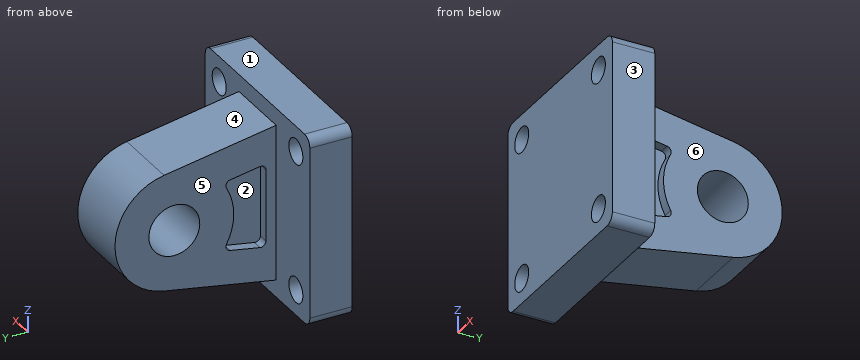
```python
from build123d import *

# Parameters (mm, degrees)
SKETCH_3_W               = 45
SKETCH_3_H               = 45
EXTRUDE_1_DEPTH          = 10
EXTRUDE_START            = -8
EXTRUDE_2_DEPTH          = 16
SKETCH_5_R               = 6
CUT_EXTRUDE_1_DEPTH      = 62.159627206
CUT_EXTRUDE_START        = -2.4
CUT_EXTRUDE_3_DEPTH      = 2.4
SKETCH_7_R               = 3
CUT_EXTRUDE_2_DEPTH      = 50.563091106
MIRROR_2_COPY_1_SKETCH_R = 3
MIRROR_2_COPY_1_DEPTH    = 50.563091106
FILLET_1_R               = 2.25
FILLET_2_R               = 1.2


with BuildPart() as part:
    # 草图3 → 凸台-拉伸1 (new body)
    with BuildSketch(Plane(origin=(0, 0, 0), x_dir=(1, 0, 0), z_dir=(0, 1, 0))):
        Rectangle(SKETCH_3_W, SKETCH_3_H)
    extrude(amount=EXTRUDE_1_DEPTH)

    # 草图4 → 凸台-拉伸2 (add)
    with BuildSketch(Plane(origin=(0, 0, 0), x_dir=(0, 0, -1), z_dir=(1, 0, 0)).offset(EXTRUDE_START)):
        with BuildLine():
            Line((-13.787308542, 36.431074487), (-18.447820103, 10))
            Line((-18.447820103, 10), (18.447820103, 10))
            Line((18.447820103, 10), (13.787308542, 36.431074487))
            ThreePointArc((13.787308542, 36.431074487), (0, 48), (-13.787308542, 36.431074487))
        make_face()
    extrude(amount=EXTRUDE_2_DEPTH)

    # 草图5 → 切除-拉伸1 (cut, through all)
    with BuildSketch(Plane(origin=(8, 0, 0), x_dir=(0, 0, -1), z_dir=(1, 0, 0))):
        with Locations((0, 34)):
            Circle(SKETCH_5_R)
    extrude(amount=-CUT_EXTRUDE_1_DEPTH, mode=Mode.SUBTRACT)

    # 草图8 → 切除-拉伸3 (cut)
    with BuildSketch(Plane(origin=(8, 0, 0), x_dir=(0, 0, -1), z_dir=(1, 0, 0)).offset(CUT_EXTRUDE_START)):
        with BuildLine():
            Line((-8.10534153, 22.584946838), (-9.901222455, 12.4))
            Line((-9.901222455, 12.4), (9.901222455, 12.4))
            Line((9.901222455, 12.4), (8.10534153, 22.584946838))
            ThreePointArc((8.10534153, 22.584946838), (0, 20), (-8.10534153, 22.584946838))
        make_face()
    cut_extrude_3 = extrude(amount=CUT_EXTRUDE_3_DEPTH, mode=Mode.SUBTRACT)

    # 镜向3: 切除-拉伸3 across plane
    add(cut_extrude_3.mirror(Plane(origin=(0, 0, 0), x_dir=(0, 0, 1), z_dir=(1, 0, 0))), mode=Mode.SUBTRACT)

    # 草图7 → 切除-拉伸2 (cut, through all)
    with BuildSketch(Plane(origin=(0, 10, 0), x_dir=(1, 0, 0), z_dir=(0, 1, 0))):
        with Locations(Location((-16.5, 16.5, 0), (0, 0, 270))):
            Circle(SKETCH_7_R)
    cut_extrude_2 = extrude(amount=-CUT_EXTRUDE_2_DEPTH, mode=Mode.SUBTRACT)

    # 镜向1: 切除-拉伸2 across plane
    add(cut_extrude_2.mirror(Plane(origin=(0, 0, 0), x_dir=(0, 0, 1), z_dir=(1, 0, 0))), mode=Mode.SUBTRACT)

    # 镜向2: 切除-拉伸2 across plane
    add(cut_extrude_2.mirror(Plane.XY), mode=Mode.SUBTRACT)

    # 镜向2 copy 1 sketch → 镜向2 copy 1 (cut, through all)
    with BuildSketch(Plane(origin=(0, 10, 0), x_dir=(-1, 0, 0), z_dir=(0, 1, 0))):
        with Locations(Location((-16.5, 16.5, 0), (0, 0, 270))):
            Circle(MIRROR_2_COPY_1_SKETCH_R)
    extrude(amount=-MIRROR_2_COPY_1_DEPTH, mode=Mode.SUBTRACT)

    # 圆角1
    fillet_1_edges = [part.edges().sort_by_distance(p)[0] for p in [
        (-22.5, 5, 22.5),
        (-22.5, 5, -22.5),
        (22.5, 5, -22.5),
        (22.5, 5, 22.5),
    ]]
    fillet(fillet_1_edges, radius=FILLET_1_R)

    # 圆角2
    fillet_2_edges = [part.edges().sort_by_distance(p)[0] for p in [
        (6.8, 22.584946838, 8.10534153),
        (6.8, 22.584946838, -8.10534153),
        (6.8, 12.4, -9.901222455),
        (6.8, 12.4, 9.901222455),
        (-6.8, 22.584946838, -8.10534153),
        (-6.8, 22.584946838, 8.10534153),
        (-6.8, 12.4, 9.901222455),
        (-6.8, 12.4, -9.901222455),
    ]]
    fillet(fillet_2_edges, radius=FILLET_2_R)


solid = part.part
```
Verification items for the finished model (mm, model axes). Face numbers are marked on the shaded views. A direction names the side the tool comes from. Give positions to 0.01 mm unless a question says otherwise; leave off trailing zeros. Order: outer loops, then holes, each group sorted by start corner. A loop starts at its lowest first (then second) coordinate and runs counter-clockwise, first axis right, second up. Notation, with made-up numbers: (81.25, -29.75) - (94.25, -29.75) arc R16 ccw to (94.25, -12.75) - close; hole circle Ø1 at (-11.75, 11.25). An arc over 180 degrees is marked (long way). Answer as CSV lines item,"result". Start each with the question number.
Item 1: Material ranges on L1, parallel to X at y = 6.25, z = 16.5; L2, parallel to Y at x = -3, z = -19, recorded low to high.
Item 2: Section check A-A, the plane x = 16.5. Record the boundary of the cut face in (y, z), plus the area to 3 significant figures.
Item 3: Mould release check, pull along Z, two halves, no side actions. Record for the marked faces 1, 2 and 3: released by +Z, released by -Z, zero draft, split by the parting line, or undercut.
Item 4: Section check D-D, the plane z = -16.5. Record the boundary of the cut face in (x, y).
Item 5: Gauge pin test, flat ends, axial feed: pin 1 (7.5 mm diameter, centred on y = 16, z = 3, fed in from +X); pin 2 (1.9 mm diameter, centred on x = -6.5, z = 1.5, fed in from +Y); pin 3 (1.5 mm diameter, centred on x = -1, y = 25.5, fed in from -Z). Record the tip position at first contact, or that the pin passes through.
Item 6: Section check C-C, the plane x = 7. Record the boundary of the cut face in (y, z), plus the area to 3 significant figures.
Item 7: Section check B-B, the plane y = 7.5. Record the boundary of the cut face in (x, z).
Item 8: Access from +Z, -Z, +X, -X, +Y, -Y to the whole of each face (thin tool, end or side, straight path). Record for the marked faces 4, 5 and 6.
Filled in:
1,L1,"-22.5 to -19.5, -13.5 to 13.5, 19.5 to 22.5"
1,L2,"0 to 10"
2,outline,"(0, -22.5) - (10, -22.5) - (10, -19.5) - (0, -19.5) - close; (0, -13.5) - (10, -13.5) - (10, 13.5) - (0, 13.5) - close; (0, 19.5) - (10, 19.5) - (10, 22.5) - (0, 22.5) - close"
2,area,"330 mm^2"
3,face 1,"released by +Z"
3,face 2,"undercut"
3,face 3,"zero draft"
4,outline,"(-22.5, 0) - (-19.5, 0) - (-19.5, 10) - (-22.5, 10) - close; (-13.5, 0) - (13.5, 0) - (13.5, 10) - (8, 10) - (8, 21.05) - (-8, 21.05) - (-8, 10) - (-13.5, 10) - close; (19.5, 0) - (22.5, 0) - (22.5, 10) - (19.5, 10) - close"
5,pin 1,"x = 8"
5,pin 2,"y = 47.99"
5,pin 3,"z = -15.85"
6,outline,"(0, -22.5) - (10, -22.5) - (10, -18.45) - (36.43, -13.79) arc R14 ccw to (36.43, 13.79) - (10, 18.45) - (10, 22.5) - (0, 22.5) - close; hole (12.4, -8.47) arc R1.2 ccw to (13.81, -9.65) - (20.84, -8.41) arc R1.2 ccw to (21.69, -6.66) arc R14 cw to (21.69, 6.66) arc R1.2 ccw to (20.84, 8.41) - (13.81, 9.65) arc R1.2 ccw to (12.4, 8.47) - close; hole circle Ø12 at (34, 0)"
6,area,"1,280 mm^2"
7,outline,"(-22.5, -20.25) arc R2.25 ccw to (-20.25, -22.5) - (20.25, -22.5) arc R2.25 ccw to (22.5, -20.25) - (22.5, 20.25) arc R2.25 ccw to (20.25, 22.5) - (-20.25, 22.5) arc R2.25 ccw to (-22.5, 20.25) - close; hole circle Ø6 at (-16.5, -16.5); hole circle Ø6 at (-16.5, 16.5); hole circle Ø6 at (16.5, -16.5); hole circle Ø6 at (16.5, 16.5)"
8,face 4,"+Z, +X, -X, +Y"
8,face 5,"+Z, -Z, -X, +Y"
8,face 6,"+Z, -Z, +X, +Y"
